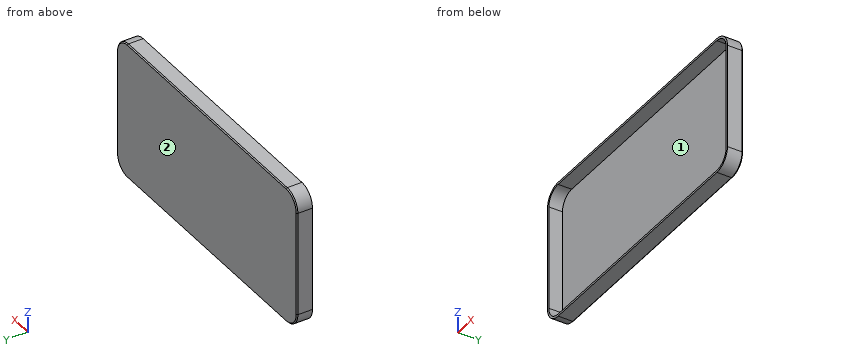
```python
from build123d import *

# Parameters (mm, degrees)
F1_DEPTH = 1
F3_DEPTH = 7.5
F5_DEPTH = 6.5
F6_SIZE  = 0.5


with BuildPart() as f1:
    # F0 (on Front) → F1 (new body)
    with BuildSketch(Plane.XZ):
        with BuildLine():
            ThreePointArc((0, 5), (1.464466, 1.464466), (5, 0))
            Line((5, 0), (125, 0))
            ThreePointArc((125, 0), (128.535534, 1.464466), (130, 5))
            Line((130, 5), (130, 55))
            ThreePointArc((130, 55), (128.535534, 58.535534), (125, 60))
            Line((125, 60), (5, 60))
            ThreePointArc((5, 60), (1.464466, 58.535534), (0, 55))
            Line((0, 55), (0, 5))
        make_face()
    extrude(amount=F1_DEPTH)

    # F2 (on face) → F3 (join)
    with BuildSketch(Plane(origin=(0, 0, 0), x_dir=(-1, 0, 0), z_dir=(0, 1, 0))):
        with BuildLine():
            ThreePointArc((3, 55), (0.656854, 60.656854), (-5, 63))
            Line((-5, 63), (-125, 63))
            ThreePointArc((-125, 63), (-130.656854, 60.656854), (-133, 55))
            Line((-133, 55), (-133, 5))
            ThreePointArc((-133, 5), (-130.656854, -0.656854), (-125, -3))
            Line((-125, -3), (-5, -3))
            ThreePointArc((-5, -3), (0.656854, -0.656854), (3, 5))
            Line((3, 5), (3, 55))
        make_face()
        with BuildLine():
            Line((0, 55), (0, 5))
            ThreePointArc((0, 5), (-1.464466, 1.464466), (-5, 0))
            Line((-5, 0), (-125, 0))
            ThreePointArc((-125, 0), (-128.535534, 1.464466), (-130, 5))
            Line((-130, 5), (-130, 55))
            ThreePointArc((-130, 55), (-128.535534, 58.535534), (-125, 60))
            Line((-125, 60), (-5, 60))
            ThreePointArc((-5, 60), (-1.464466, 58.535534), (0, 55))
        make_face(mode=Mode.SUBTRACT)
    extrude(amount=-F3_DEPTH)

    # F4 (on face) → F5 (cut, through all)
    with BuildSketch(Plane.XZ.offset(7.5)):
        with BuildLine():
            Line((125, 62), (5, 62))
            ThreePointArc((5, 62), (0.050253, 59.949747), (-2, 55))
            Line((-2, 55), (-2, 5))
            ThreePointArc((-2, 5), (0.050253, 0.050253), (5, -2))
            Line((5, -2), (125, -2))
            ThreePointArc((125, -2), (129.949747, 0.050253), (132, 5))
            Line((132, 5), (132, 55))
            ThreePointArc((132, 55), (129.949747, 59.949747), (125, 62))
        make_face()
        with BuildLine():
            ThreePointArc((5, 0), (1.464466, 1.464466), (0, 5))
            Line((0, 5), (0, 55))
            ThreePointArc((0, 55), (1.464466, 58.535534), (5, 60))
            Line((5, 60), (125, 60))
            ThreePointArc((125, 60), (128.535534, 58.535534), (130, 55))
            Line((130, 55), (130, 5))
            ThreePointArc((130, 5), (128.535534, 1.464466), (125, 0))
            Line((125, 0), (5, 0))
        make_face(mode=Mode.SUBTRACT)
    extrude(amount=-F5_DEPTH, mode=Mode.SUBTRACT)

    # F6
    f6_edges = [f1.edges().sort_by_distance(p)[0] for p in [
        (-0.656854, 0, -0.656854),
        (65, 0, -3),
        (130.656854, 0, -0.656854),
        (133, 0, 30),
        (130.656854, 0, 60.656854),
        (65, 0, 63),
        (-0.656854, 0, 60.656854),
        (-3, 0, 30),
    ]]
    chamfer(f6_edges, length=F6_SIZE)


solid = f1.part
```
Build history of the part. All positions in model axes, mm. Face numbers are marked on the shaded views. Coordinates: 2 decimals unless noted, no trailing zeros. Order: outer loops, then holes, each group sorted by start corner. A loop starts at its lowest first (then second) coordinate and runs counter-clockwise, first axis right, second up. Notation, with made-up numbers: (80.5, 50.5) -> (88.5, 50.5) arc R18 ccw to (88.5, 69.5) -> close; hole circle Ø8 at (-26, 40.25). An arc over 180 degrees is marked (long way). Answer in a Markdown table with one row per item. Add a question column.
Q1. Band-saw the part on A-A, the plane y = -2.5. List the corners of the cut face in (x, z), then the cut area to 3 significant figures.
Q2. Wall check: line 1 along X through (y, z) = (-1.25, 21); line 2 along Z through (x, y) = (75.5, -1.75); line 3 along Y through (x, z) = (65, 16). Give the ranges that are in metal, low to high. Write a range as [from, to].
Q3. Mould opens along X. For the marked faces 1 and 2 say: +X half, -X half, draft (parallel to the pull), parting line (faces both ways), or undercut.
Q4. Band-saw the part on C-C, the plane z = 32. List the corners of the cut face in (x, y).
Q5. Band-saw the part on B-B, the plane x = 60. List the corners of the cut face in (y, z), then the cut area to 4 significant figures.
Answers follow:
| question | item | result |
|---|---|---|
| 1 | outline | (-3, 5) arc R8 ccw to (5, -3) -> (125, -3) arc R8 ccw to (133, 5) -> (133, 55) arc R8 ccw to (125, 63) -> (5, 63) arc R8 ccw to (-3, 55) -> close; hole (-2, 5) arc R7 ccw to (5, -2) -> (125, -2) arc R7 ccw to (132, 5) -> (132, 55) arc R7 ccw to (125, 62) -> (5, 62) arc R7 ccw to (-2, 55) -> close |
| 1 | area | 387 mm^2 |
| 2 | line 1 | [-3, -2], [132, 133] |
| 2 | line 2 | [-3, -2], [62, 63] |
| 2 | line 3 | [-1, 0] |
| 3 | face 1 | undercut |
| 3 | face 2 | draft |
| 4 | outline | (-3, -7.5) -> (-2, -7.5) -> (-2, -1) -> (132, -1) -> (132, -7.5) -> (133, -7.5) -> (133, -0.5) -> (132.5, 0) -> (-2.5, 0) -> (-3, -0.5) -> close |
| 5 | outline | (-7.5, -3) -> (-0.5, -3) -> (0, -2.5) -> (0, 62.5) -> (-0.5, 63) -> (-7.5, 63) -> (-7.5, 62) -> (-1, 62) -> (-1, -2) -> (-7.5, -2) -> close |
| 5 | area | 78.75 mm^2 |
